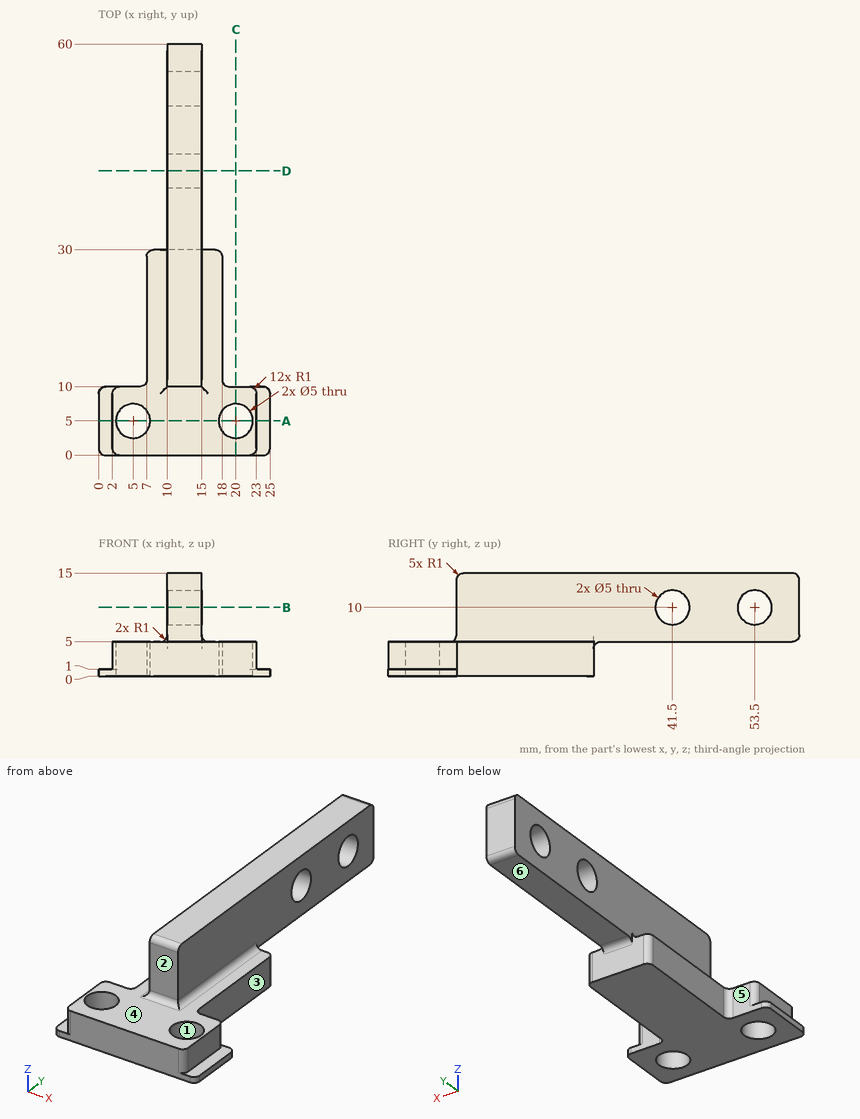
Answer from the drawing. Dimensions are ordinates in mm from the lowest x, y and z of the part. A direction names the side the tool comes from. Give positions to 0.01 mm unless a question says otherwise; leave off trailing zeros. Order: outer loops, then holes, each group sorted by start corner. A loop starts at its lowest first (then second) coordinate and runs counter-clockwise, first axis right, second up. Notation, with made-up numbers: (80, -29.75) - (117, -29.75) arc R18 ccw to (117, -12.75) - close; hole circle Ø1 at (-38, 40). An arc over 180 degrees is marked (long way). One line per item, written item: value. Start each with the question number.
1. Which of the six approach directions +Z, -Z, +X, -X, +Y, -Y give full straight-line access (tool end or side, diameter ignored) to the marked faces 4, 5 and 6?
2. For a pull along Y with two mould halves and no side action, classify the marked faces 1, 2 and 3 as released by +Y, released by -Y, zero draft, split by the parting line, or undercut.
3. Each of these flat-tipped pins is pushed along its axis until it touches: pin 1 Ø4.5 at (y, z) = (5, 3.5) entering from -X; pin 2 Ø4 at (x, z) = (2.5, 1.5) entering from +Y; pin 3 Ø1.5 at (x, z) = (12, 10.5) entering from -Y; pin 4 Ø6 at (x, y) = (4.5, 46) entering from -Z. Where does it stop, or does it pass through?
4. Section C-C, the plane x = 20 is taken. Write down the section's boundary in (y, z).
5. Consider line 1 (Y direction, x = 12.5, z = 9.75); line 2 (Y direction, x = 20, z = 2.25); line 3 (Z direction, x = 12.65, y = 41.5). Determine where each line is inside the solid, lowest interval first.
6. Section D-D, the plane y = 41.5 is taken. Write down the section's boundary in (x, z), then the cut area to 3 significant figures.
7. Section B-B, the plane z = 10 is taken. Write down the section's boundary in (x, y).
8. Section A-A, the plane y = 5 is taken. Write down the section's boundary in (x, z).
Filled sheet:
1. face 4: +Z, -Y
1. face 5: +Z, -Z, -X, +Y
1. face 6: -Z, +X, -X, +Y
2. face 1: undercut
2. face 2: released by -Y
2. face 3: zero draft
3. pin 1: x = 2
3. pin 2: y = 10
3. pin 3: y = 10
3. pin 4: through
4. outline: (0, 0) - (2.5, 0) - (2.5, 5) - (0, 5) - close; (7.5, 0) - (10, 0) - (10, 5) - (7.5, 5) - close
5. line 1: 10 to 39.01, 43.99 to 51.01, 55.99 to 60
5. line 2: 0 to 2.5, 7.5 to 10
5. line 3: 5 to 7.5, 12.5 to 15
6. outline: (10, 5) - (15, 5) - (15, 7.5) - (10, 7.5) - close; (10, 12.5) - (15, 12.5) - (15, 15) - (10, 15) - close
6. area: 25.0 mm²
7. outline: (10, 10) - (15, 10) - (15, 39) - (10, 39) - close; (10, 44) - (15, 44) - (15, 51) - (10, 51) - close; (10, 56) - (15, 56) - (15, 60) - (10, 60) - close
8. outline: (0, 0) - (2.5, 0) - (2.5, 5) - (2, 5) - (2, 1) - (0, 1) - close; (7.5, 0) - (17.5, 0) - (17.5, 5) - (7.5, 5) - close; (22.5, 0) - (25, 0) - (25, 1) - (23, 1) - (23, 5) - (22.5, 5) - close
